```python
from build123d import *

# Parameters (mm, degrees)
F0_W          = 25
F0_H          = 25
F1_DEPTH      = 150
F1_DEPTH_BACK = 150
F2_R          = 5
F5_W          = 25
F5_H          = 25
F6_DEPTH      = 300
F7_W          = 25
F7_H          = 25
F7_H_2        = 50
F8_DEPTH      = 5


with BuildPart() as f1:
    # F0 (on Right) → F1 (new body, two sides)
    with BuildSketch(Plane.YZ) as f1_sk:
        Rectangle(F0_W, F0_H)
    extrude(amount=F1_DEPTH)
    extrude(f1_sk.sketch, amount=-F1_DEPTH_BACK)

    # F4: sweep along a path in F3
    with BuildLine(Plane.YZ) as f4_path:
        Line((-12.5, 0), (-462.5, 0))
        ThreePointArc((-462.5, 0), (-477.7069063257, 1.2585620455), (-492.5, 5))
    # F2 (on face) → F4 (sweep)
    with BuildSketch(Plane.XZ.offset(12.5)):
        with Locations((-100, 0)):
            Circle(F2_R)
        with Locations((100, 0)):
            Circle(F2_R)
    sweep(path=f4_path.line)

    # F5 (on face) → F6 (join)
    with BuildSketch(Plane(origin=(0, 0, -12.5), x_dir=(1, 0, 0), z_dir=(0, 0, -1))):
        with Locations((-137.5, 0)):
            Rectangle(F5_W, F5_H)
        with Locations((137.5, 0)):
            Rectangle(F5_W, F5_H)
    extrude(amount=F6_DEPTH)

    # F7 (on face) → F8 (join)
    with BuildSketch(Plane(origin=(0, 0, -312.5), x_dir=(1, 0, 0), z_dir=(0, 0, -1))):
        with Locations((-137.5, 0)):
            Rectangle(F7_W, F7_H)
        with Locations((-137.5, -37.5)):
            Rectangle(F7_W, F7_H_2)
        with Locations((-137.5, 37.5)):
            Rectangle(F7_W, F7_H_2)
        with Locations((137.5, 0)):
            Rectangle(F7_W, F7_H)
        with Locations((137.5, 37.5)):
            Rectangle(F7_W, F7_H_2)
        with Locations((137.5, -37.5)):
            Rectangle(F7_W, F7_H_2)
    extrude(amount=F8_DEPTH)


solid = f1.part
```
Geometry: final body of the model. Coordinates: model frame, mm. A direction names the side the tool comes from. Give positions to 0.01 mm unless a question says otherwise; leave off trailing zeros. Write each loop counter-clockwise with the first axis right and the second up, starting at its lowest first coordinate (ties: lowest second). Pieces come first, ordered by that corner, then holes.
1. Line query: probe 1 along X at (y, z) = (3.5, -283); probe 2 along Y at (x, z) = (131.5, -248); probe 3 along Z at (x, y) = (-101, -264.5). Output: solid intervals per line, ascending.
2. Section query A-A, the plane z = -48.5. Return loops of the section in (x, y).
3. Section query C-C, the plane y = -178. Return loops of the section in (x, z), then the cut area to 3 significant figures.
4. Section query D-D, the plane x = -42. Return loops of the section in (y, z), then the cut area to 3 significant figures.
5. Section query B-B, the plane y = -51. Return loops of the section in (x, z), then the cut area to 3 significant figures.
6. Pin query (flat end, axial travel): P1, Ø7.5, axis at x = -136, y = -43, coming from the +Z side; P2, Ø1.5, axis at x = -132, z = -315.5, coming from the -Y side. Return the tip coordinate at first contact, or that it passes through.
7. Draft query along X for faces 6 (the flat face through (-23, 12.5, -5)), 7 (the flat face through (125, 0, -164)), 8 (the flat face through (-150, 0, -152)). Return one class per face: released by +X, released by -X, zero draft, split by the parting line, or undercut.
8. Reachability of faces 1 (the flat face through (2, 0, 12.5)), 2 (the flat face through (-125, 0, -164)), 3 (the flat face through (137, -1, -317.5)), 4 (the flat face through (-138, -38, -312.5)), 5 (the flat face through (-138, 37, -312.5)) from +Z, -Z, +X, -X, +Y, -Y: full face, straight path, thin tool, end or side. Return the list, or none.
Computed:
1. probe 1: x = -150 to -125, 125 to 150
1. probe 2: y = -12.5 to 12.5
1. probe 3: z = -4.9 to 4.9
2. outline: (-150, -12.5) - (-125, -12.5) - (-125, 12.5) - (-150, 12.5) - close; (125, -12.5) - (150, -12.5) - (150, 12.5) - (125, 12.5) - close
3. outline: circle Ø10 at (-100, 0); circle Ø10 at (100, 0)
3. area: 157 mm2
4. outline: (-12.5, -12.5) - (12.5, -12.5) - (12.5, 12.5) - (-12.5, 12.5) - close
4. area: 625 mm2
5. outline: (-150, -317.5) - (-125, -317.5) - (-125, -312.5) - (-150, -312.5) - close; circle Ø10 at (-100, 0); circle Ø10 at (100, 0); (125, -317.5) - (150, -317.5) - (150, -312.5) - (125, -312.5) - close
5. area: 407 mm2
6. P1: stops at z = -312.5
6. P2: stops at y = -62.5
7. face 6: zero draft
7. face 7: undercut
7. face 8: released by -X
8. face 1: +Z, +X, -X, +Y, -Y
8. face 2: -Z, +Y, -Y
8. face 3: -Z, +X, -X, +Y, -Y
8. face 4: +Z, +X, -X, -Y
8. face 5: +Z, +X, -X, +Y
